Autodesk Inventor part; units mm, degrees
ref_plane "YZ Plane" through (0, 0, 0) normal (1, 0, 0) x (0, 1, 0)
ref_plane "XZ Plane" through (0, 0, 0) normal (0, 1, 0) x (-1, 0, 0)
ref_plane "XY Plane" through (0, 0, 0) normal (0, 0, 1) x (1, 0, 0)
sketch "Boceto1" plane through (0, 0, 0) normal (0, 0, 1) x (1, 0, 0)
  arc A0 (-14.2261, 5.0309) -> (-14.2261, 1.0422) centre (-14.0761, 3.0366) ccw
  line L0 (-14.2261, 5.0309) -> (-0.0106, 6.0724)
  line L1 (-14.2261, 1.0422) -> (0, 0)
  circle A1 centre (-14.6761, 3.0366) radius 0.5
  circle A2 centre (-12.6761, 3.0366) radius 0.5
  circle A3 centre (-10.6761, 3.0366) radius 0.5
  circle A4 centre (-8.6761, 3.0366) radius 0.5
  circle A5 centre (-6.6761, 3.0366) radius 0.5
  circle A6 centre (-4.6761, 3.0366) radius 0.5
  line L2 (-0.2768, 6.0529) -> (0, 6.0731)
  arc A7 (14.2261, 1.0422) -> (14.2264, 5.0339) centre (14.0972, 3.038) ccw
  line L3 (14.2264, 5.0339) -> (0.0108, 6.0753)
  line L4 (14.2261, 1.0422) -> (0, 0)
  circle A8 centre (14.6761, 3.0366) radius 0.5
  circle A9 centre (12.6761, 3.0366) radius 0.5
  circle A10 centre (10.6761, 3.0366) radius 0.5
  circle A11 centre (8.6761, 3.0366) radius 0.5
  circle A12 centre (6.6761, 3.0366) radius 0.5
  circle A13 centre (4.6761, 3.0366) radius 0.5
  line L5 (0, 6.0731) -> (0.0201, 6.0746)
  point P0 (0, 0)
  dimension "d10" = 2
  dimension "d13" = 10
extrude "Extrusión1" add sketch "Boceto1" along normal blind 1.6
sketch "Boceto2" plane through (0, 0, 0) normal (0, 0, -1) x (-1, 0, 0)
  line L0 (0, 0) -> (-14.2261, 1.0422)
  circle A0 centre (0, 3.0373) radius 3.58
  point P0 (-0.0201, 6.0746)
extrude "Extrusión2" add sketch "Boceto2" against normal blind 3.43
sketch "Boceto3" plane through (0, 0, 0) normal (0, 0, -1) x (-1, 0, 0)
  arc A0 (2.1264, 5.9174) -> (-2.122, 5.9206) centre (0, 3.0373) ccw
  circle A1 centre (0, 3.0373) radius 2.425
  point P0 (0, 0)
extrude "Extrusión3" cut sketch "Boceto3" against normal blind 0.63
sketch "Boceto4" plane through (0, 3.0373, 0.63) normal (0, 0, -1) x (-1, 0, 0)
  circle A0 centre (0, 0) radius 0.85
  point P0 (0, -3.0373)
extrude "Extrusión4" cut sketch "Boceto4" against normal through all
sketch "Boceto5" plane through (0, 3.0373, 3.43) normal (0, 0, 1) x (1, 0, 0)
  circle A0 centre (0, 0) radius 2.3
  point P0 (0, -3.0373)
extrude "Extrusión5" cut sketch "Boceto5" against normal blind 1.83
equation "\"Radio_pliegue\" = Grosor"
equation "\"Anchura_desahogo_plegado\" = Grosor"
equation "\"Profundidad_desahogo_plegado\" = 0.5 * Grosor"
equation "\"Tamaño_destalonado\" = 4 * Grosor"
equation "\"Remanente_mínimo\" = 2 * Grosor"
equation "\"Radiodetransición\" = Radio_pliegue"
equation "\"Tamaño_de_radio_de_Jacobi\" = Radio_pliegue"
equation "\"TamañoSeparación\" = Grosor"
properties part number "cosito servo"
For this review, take the finished solid that the model builds, in its own axes (mm). A direction names the side the tool comes from. Round coordinates to 2 decimals unless told otherwise and drop trailing zeros. Order: outer loops, then holes, each group sorted by start corner. A loop starts at its lowest first (then second) coordinate and runs counter-clockwise, first axis right, second up. Notation, with made-up numbers: M -17,13 L -12,13 A22 cw -12,33 Z; hole C -5.5,12.25 d1. An arc over 180 degrees is marked long. Use a Markdown table: item, result. Add a question column.
Item 1: Add section B-B, the plane z = 2.9. Give the boundary of the cut face in (x, y), then the cut area to 3 significant figures.
Item 2: Add section A-A, the plane z = 0.95. State how many separate pieces and enclosed holes the cut face has, then the cut area to 3 significant figures.
Item 3: Insertion check: pin 1 (3 mm diameter, centred on x = -11, y = 4.5, fed in from +Z); pin 2 (2 mm diameter, centred on x = -9.5, z = 1.5, fed in from -Y); pin 3 (1 mm diameter, centred on y = 4, z = 1, fed in from -X). Each pin has a flat end and moves straight along its axis. Give the tip position at first contact, or say it passes through.
Item 4: Mouldability with a two-part tool opening along X and no side actions: class faces 1 (the flat face through (-9, 2, 1.6)), 2 (the cylindrical face through (-16.076, 2.995, 0.789)), 3 (the cylindrical face through (6.308, 2.699, 0.789)) as released by +X, released by -X, zero draft, split by the parting line, or undercut.
Item 5: Add section C-C, the plane x = 1.5. Give the boundary of the cut face in (y, z).
Item 6: To check wall thickness, follow line 1 along Z through (x, y) = (7, 5.5); line 2 along Y through (x, z) = (0, 1); line 3 along X through (y, z) = (1.25, 3.25). State the ranges of each line that lie inside material, in increasing order.
Item 7: Add section D-D, the plane y = 1.5. Give the boundary of the cut face in (x, z), then the cut area to 3 significant figures.
Item 8: Tool access review of faces 4 (the cylindrical face through (0.11, 3.88, 1.11)), 5 (the cylindrical face through (-0.499, 0.792, 2.528)), 6 (the cylindrical face through (-1.304, 5.082, 0.311)): name each direction out of +Z, -Z, +X, -X, +Y, -Y from which nothing blocks a thin tool from reaching the whole face with its end or side.
Geometry results:
| question | item | result |
|---|---|---|
| 1 | outline | C 0,3.04 d7.16; hole C 0,3.04 d4.6 |
| 1 | area | 23.6 mm² |
| 2 | separate pieces | 1 |
| 2 | enclosed holes | 13 |
| 2 | area | 146 mm² |
| 3 | pin 1 | stops at z = 1.6 |
| 3 | pin 2 | stops at y = 0.62 |
| 3 | pin 3 | stops at x = -16.02 |
| 4 | face 1 | zero draft |
| 4 | face 2 | released by -X |
| 4 | face 3 | undercut |
| 5 | outline | M -0.21,0 L 1.13,0 L 1.13,0.63 L 4.94,0.63 L 4.94,0 L 6.29,0 L 6.29,3.43 L 4.78,3.43 L 4.78,1.6 L 1.29,1.6 L 1.29,3.43 L -0.21,3.43 Z |
| 6 | line 1 | z = 0 to 1.6 |
| 6 | line 2 | y = -0.54 to 2.19, 3.89 to 6.62 |
| 6 | line 3 | x = -3.1 to -1.45, 1.45 to 3.1 |
| 7 | outline | M -15.36,0 L -1.88,0 L -1.88,0.63 L 1.88,0.63 L 1.88,0 L 15.38,0 L 15.38,1.6 L 3.23,1.6 L 3.23,3.43 L 1.71,3.43 L 1.71,1.6 L -1.71,1.6 L -1.71,3.43 L -3.23,3.43 L -3.23,1.6 L -15.36,1.6 Z |
| 7 | area | 52.4 mm² |
| 8 | face 4 | +Z, -Z |
| 8 | face 5 | +Z |
| 8 | face 6 | -Z |
